Can you work these out from the model? Positions are in its coordinate system, mm. A direction names the side the tool comes from. Give positions to 0.01 mm unless a question says otherwise; leave off trailing zeros. Write each loop counter-clockwise with the first axis right and the second up, starting at its lowest first coordinate (ties: lowest second). Pieces come first, ordered by that corner, then holes. Notation, with made-up numbers: (15, 53) - (37, 53) arc R15 ccw to (37, 69) - close; hole circle Ø9 at (35, 63.25). An arc over 180 degrees is marked (long way). Use a Markdown table: item, result. Add a question column.
Autodesk Inventor part; units mm, degrees
ref_plane "YZ Plane" through (0, 0, 0) normal (1, 0, 0) x (0, 1, 0)
ref_plane "XZ Plane" through (0, 0, 0) normal (0, 1, 0) x (-1, 0, 0)
ref_plane "XY Plane" through (0, 0, 0) normal (0, 0, 1) x (1, 0, 0)
sketch "Sketch1" plane through (0, 0, 0) normal (0, 1, 0) x (-1, 0, 0)
  line L0 (0, 0) -> (-86, 0)
  line L1 (-86, 0) -> (-86, -157)
  line L2 (-86, -157) -> (0, -157)
  line L3 (0, -157) -> (0, 0)
  line L4 (-14, -40) -> (-46, -40) construction
  line L5 (-46, -40) -> (-46, -10) construction
  line L6 (-46, -10) -> (-14, -10) construction
  line L7 (-14, -10) -> (-14, -40) construction
  line L8 (-14, -147) -> (-46, -147) construction
  line L9 (-46, -147) -> (-46, -117) construction
  line L10 (-46, -117) -> (-14, -117) construction
  line L11 (-14, -117) -> (-14, -147) construction
  line L12 (-86, -110) -> (-61, -110)
  line L13 (-61, -110) -> (-61, -108.3)
  line L14 (-61, -108.3) -> (-86, -108.3)
  line L15 (-86, -48.7) -> (-61, -48.7)
  line L16 (-61, -48.7) -> (-61, -47)
  line L17 (-61, -47) -> (-86, -47)
  line L18 (-20, -57) -> (-39.9, -57) construction
  dimension "d0" = 86
  dimension "d1" = 157
  dimension "d2" = 32
  dimension "d3" = 30
  dimension "d4" = 14
  dimension "d5" = 10
  dimension "d6" = 32
  dimension "d7" = 30
  dimension "d8" = 10
  dimension "d9" = 14
  dimension "d10" = 1.7
  dimension "d11" = 1.7
  dimension "d13" = 47
  dimension "d15" = 25
  dimension "d16" = 47
  dimension "d26" = 19.9
  dimension "d27" = 20
  dimension "d28" = 57
extrude "Extrusion1" add sketch "Sketch1" along normal blind 3 contours L3 L2 L1 L12 L13 L14 L15 L16 L17 L0
hole "Hole1" at (14, 0, -40) at (46, 0, -40) at (46, 0, -10) at (14, 0, -10) at (14, 0, -147) at (46, 0, -117) at (14, 0, -117) at (46, 0, -147) direction (0, 1, 0) diameter 5 end through all
hole "Hole2" at (20, 0, -57) at (39.9, 0, -57) direction (0, 1, 0) diameter 4 end through all
properties part number "X Axis Base Plate Accurate_3DPrint"
Q1. If I drill on probe 1 along Z at (x, y) = (14, 1.1); probe 2 along X at (y, z) = (0.95, -40); probe 3 along Z at (x, y) = (82, 0.75), over which ranges is the centre line in solid material (lowest first)? Write a range as [from, to].
Q2. Suppose I cut it at C-C (y = 0.5). Give the number of separate pieces and of enclosed holes in the cut face, and give its area (3 significant figures).
Q3. Suppose I cut it at A-A (x = 20). Please give me the cut outline in (y, z), and give its area (3 significant figures).
Q4. On a 3-axis mill with a long thin cutter (end or side, diameter ignored), from which of +Z, -Z, +X, -X, +Y, -Y can I reach the whole of each face in a straight line? I mean faces 1 (the flat face through (86, 1, -23)), 2 (the flat face through (73, 1, -47)). Say none if no direction works.
Q5. Suppose I cut it at B-B (z = -147). Please give me the cut outline in (x, y), and give its area (3 significant figures).
Q6. If we mould it in two halves opening along Z, with no side actions, what happens to faces 3 (the cylindrical face through (16.44, 1.52, -9.46)), 4 (the flat face through (42, 1, 0)), 5 (the flat face through (0, 1, -80))? For each: released by +Z, released by -Z, zero draft, split by the parting line, or undercut.
Q7. I'm going to push flat-ended pins straight in: P1, Ø0.5, axis at y = 1.5, z = -48, coming from the +X side; P2, Ø2.5, axis at x = 39.9, z = -57, coming from the +Y side. Where does each tip first touch, or does it pass through?
Derived:
| question | item | result |
|---|---|---|
| 1 | probe 1 | [-157, -149.5], [-144.5, -119.5], [-114.5, -42.5], [-37.5, -12.5], [-7.5, 0] |
| 1 | probe 2 | [0, 11.5], [16.5, 43.5], [48.5, 86] |
| 1 | probe 3 | [-157, -110], [-108.3, -48.7], [-47, 0] |
| 2 | separate pieces | 1 |
| 2 | enclosed holes | 10 |
| 2 | area | 13,200 mm² |
| 3 | outline | (0, -157) - (3, -157) - (3, -59) - (0, -59) - close; (0, -55) - (3, -55) - (3, 0) - (0, 0) - close |
| 3 | area | 459 mm² |
| 4 | face 1 | +Z, -Z, +X, +Y, -Y |
| 4 | face 2 | +X, +Y, -Y |
| 5 | outline | (0, 0) - (11.5, 0) - (11.5, 3) - (0, 3) - close; (16.5, 0) - (43.5, 0) - (43.5, 3) - (16.5, 3) - close; (48.5, 0) - (86, 0) - (86, 3) - (48.5, 3) - close |
| 5 | area | 228 mm² |
| 6 | face 3 | undercut |
| 6 | face 4 | released by +Z |
| 6 | face 5 | zero draft |
| 7 | P1 | x = 61 |
| 7 | P2 | through |
